CAD build for the part. Positions are in the model's coordinates, mm. Give positions to 0.01 mm unless a question says otherwise; leave off trailing zeros. Write each loop counter-clockwise with the first axis right and the second up, starting at its lowest first coordinate (ties: lowest second). Pieces come first, ordered by that corner, then holes. Notation, with made-up numbers: (39.25, -29.5) - (57.25, -29.5) arc R30 cw to (57.25, 2.5) - close; hole circle Ø6 at (48, 14.5). An arc over 180 degrees is marked (long way). Put each result on its own line as item: value. Start each with the question number.
1. Cut at D-D on x = 29. List the corners of the cut face in (y, z), and give its area (3 significant figures).
2. Mould opens along X. For faces 1 (the flat face through (1, 0, 10)), 2 (the cylindrical face through (14.418, 1.479, 45.783)), 3 (the cylindrical face through (-19.922, 1.521, -0.338)) say: +X half, -X half, draft (parallel to the pull), parting line (faces both ways), or undercut.
3. Drop flat-ended pins along their axis: pin 1 (1.5 mm diameter, centred on x = -1, y = 1.5, fed in from +Z); pin 2 (1.5 mm diameter, centred on y = 1.5, z = 36, fed in from -X). Give the stop position or say it passes through.
4. Wall check: line 1 (X direction, y = 0.7, z = 0); line 2 (X direction, y = 1.9, z = -26); line 3 (X direction, y = 1.45, z = -29). Give the ranges that are in metal, low to high.
5. Cut at C-C on y = 0.55. Give the number of separate pieces and of enclosed holes in the cut face, and give its area (3 significant figures).
6. Cut at B-B on x = 0. List the corners of the cut face in (y, z), and give its area (3 significant figures).
7. Cut at A-A on z = 0. List the corners of the cut face in (x, y).
from build123d import *

# Parameters (mm, degrees)
SKETCH_1_R          = 48
SKETCH_1_R_2        = 2.1
EXTRUDE_1_DEPTH     = 3
SKETCH_2_R          = 7
SKETCH_2_R_2        = 2.6
CUT_EXTRUDE_1_DEPTH = 68.948509917
SKETCH_3_R          = 1.5
CUT_EXTRUDE_2_DEPTH = 10


with BuildPart() as part:
    # 草图1 → 凸台-拉伸1 (new body)
    with BuildSketch(Plane(origin=(0, 0, 0), x_dir=(1, 0, 0), z_dir=(0, 1, 0))):
        with Locations(Location((0, 0, 0), (0, 0, 270))):
            Circle(SKETCH_1_R)
        with Locations(Location((-29, 29, 0), (0, 0, 270))):
            Circle(SKETCH_1_R_2, mode=Mode.SUBTRACT)
        with Locations(Location((29, 29, 0), (0, 0, 270))):
            Circle(SKETCH_1_R_2, mode=Mode.SUBTRACT)
        with Locations(Location((29, -29, 0), (0, 0, 270))):
            Circle(SKETCH_1_R_2, mode=Mode.SUBTRACT)
        with Locations(Location((-29, -29, 0), (0, 0, 270))):
            Circle(SKETCH_1_R_2, mode=Mode.SUBTRACT)
    extrude(amount=EXTRUDE_1_DEPTH)

    # 草图2 → 切除-拉伸1 (cut, through all)
    with BuildSketch(Plane(origin=(0, 3, 0), x_dir=(1, 0, 0), z_dir=(0, 1, 0))):
        with Locations(Location((0, 0, 0), (0, 0, 270))):
            Circle(SKETCH_2_R)
        with Locations(Location((-22.5, 0, 0), (0, 0, 270))):
            Circle(SKETCH_2_R_2)
        with Locations(Location((22.5, 0, 0), (0, 0, 270))):
            Circle(SKETCH_2_R_2)
    extrude(amount=-CUT_EXTRUDE_1_DEPTH, mode=Mode.SUBTRACT)

    # 草图3 → 切除-拉伸2 (cut)
    with BuildSketch(Plane(origin=(0, 3, 0), x_dir=(1, 0, 0), z_dir=(0, 1, 0))):
        with Locations(Location((4, 26, 0), (0, 0, 270))):
            Circle(SKETCH_3_R)
        with Locations(Location((-4, 26, 0), (0, 0, 270))):
            Circle(SKETCH_3_R)
        with Locations(Location((-4, -26, 0), (0, 0, 270))):
            Circle(SKETCH_3_R)
        with Locations(Location((4, -26, 0), (0, 0, 270))):
            Circle(SKETCH_3_R)
    extrude(amount=-CUT_EXTRUDE_2_DEPTH, mode=Mode.SUBTRACT)


solid = part.part
Report:
1. outline: (0, -38.25) - (3, -38.25) - (3, -31.1) - (0, -31.1) - close; (0, -26.9) - (3, -26.9) - (3, 26.9) - (0, 26.9) - close; (0, 31.1) - (3, 31.1) - (3, 38.25) - (0, 38.25) - close
1. area: 204 mm²
2. face 1: draft
2. face 2: parting line
2. face 3: undercut
3. pin 1: stops at z = 48
3. pin 2: stops at x = -32.58
4. line 1: x = -48 to -25.1, -19.9 to -7, 7 to 19.9, 25.1 to 48
4. line 2: x = -40.35 to -5.5, -2.5 to 2.5, 5.5 to 40.35
4. line 3: x = -38.25 to -31.1, -26.9 to 26.9, 31.1 to 38.25
5. separate pieces: 1
5. enclosed holes: 11
5. area: 6,960 mm²
6. outline: (0, -48) - (3, -48) - (3, -7) - (0, -7) - close; (0, 7) - (3, 7) - (3, 48) - (0, 48) - close
6. area: 246 mm²
7. outline: (-48, 0) - (-25.1, 0) - (-25.1, 3) - (-48, 3) - close; (-19.9, 0) - (-7, 0) - (-7, 3) - (-19.9, 3) - close; (7, 0) - (19.9, 0) - (19.9, 3) - (7, 3) - close; (25.1, 0) - (48, 0) - (48, 3) - (25.1, 3) - close
